Geometry: final body of the model. Coordinates: model frame, mm. Face numbers are marked on the shaded views. A direction names the side the tool comes from. Give positions to 0.01 mm unless a question says otherwise; leave off trailing zeros. Write each loop counter-clockwise with the first axis right and the second up, starting at its lowest first coordinate (ties: lowest second). Pieces come first, ordered by that corner, then holes. Notation, with made-up numbers: M 85,-23 L 141,-23 A18 ccw 141,-14 Z; hole C 17,35 d10. An arc over 180 degrees is marked long. One line per question, with ' | ' between items.
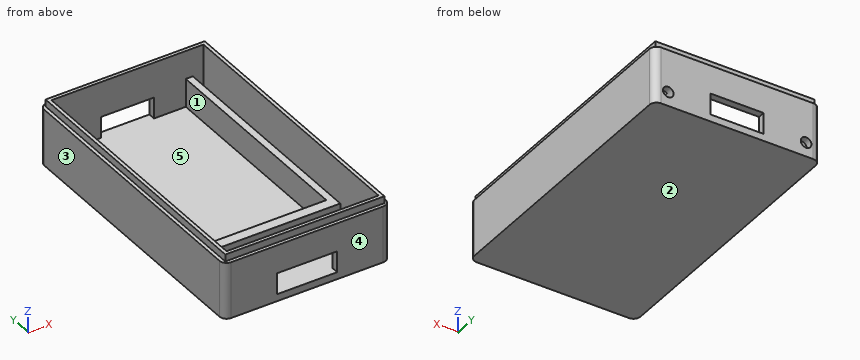
from build123d import *

# Parameters (mm, degrees)
SKETCH1_W           = 47
SKETCH1_H           = 80
BOSS_EXTRUDE1_DEPTH = 18
SKETCH2_W           = 43
SKETCH2_H           = 76
CUT_EXTRUDE1_DEPTH  = 16
BOSS_EXTRUDE2_DEPTH = 8
SKETCH6_W           = 15
SKETCH6_H           = 6
CUT_EXTRUDE4_DEPTH  = 11
SKETCH8_W           = 47
SKETCH8_H           = 80
SKETCH8_W_2         = 45
SKETCH8_H_2         = 78
CUT_EXTRUDE5_DEPTH  = 2
SKETCH9_R           = 1.5
CUT_EXTRUDE6_DEPTH  = 10
SKETCH11_W          = 17
SKETCH11_H          = 6
CUT_EXTRUDE9_DEPTH  = 10
FILLET4_R           = 2


with BuildPart() as part:
    # Sketch1 → Boss-Extrude1 (new body)
    with BuildSketch(Plane.XY):
        Rectangle(SKETCH1_W, SKETCH1_H)
    extrude(amount=BOSS_EXTRUDE1_DEPTH)

    # Sketch2 → Cut-Extrude1 (cut)
    with BuildSketch(Plane.XY.offset(18)):
        Rectangle(SKETCH2_W, SKETCH2_H)
    extrude(amount=-CUT_EXTRUDE1_DEPTH, mode=Mode.SUBTRACT)

    # Sketch3 → Boss-Extrude2 (add)
    with BuildSketch(Plane.XY.offset(2)):
        Polygon((-18.5, 38), (-16.5, 38), (-16.5, -23), (16.5, -23), (16.5, 38), (18.5, 38), (18.5, -26), (-18.5, -26), align=None)
    extrude(amount=BOSS_EXTRUDE2_DEPTH)

    # Sketch6 → Cut-Extrude4 (cut)
    with BuildSketch(Plane.XZ.offset(-38)):
        with Locations((0, 5)):
            Rectangle(SKETCH6_W, SKETCH6_H)
    extrude(amount=-CUT_EXTRUDE4_DEPTH, mode=Mode.SUBTRACT)

    # Sketch8 → Cut-Extrude5 (cut)
    with BuildSketch(Plane.XY.offset(18)):
        Rectangle(SKETCH8_W, SKETCH8_H)
        Rectangle(SKETCH8_W_2, SKETCH8_H_2, mode=Mode.SUBTRACT)
    extrude(amount=-CUT_EXTRUDE5_DEPTH, mode=Mode.SUBTRACT)

    # Sketch9 → Cut-Extrude6 (cut)
    with BuildSketch(Plane(origin=(0, 40, 0), x_dir=(1, 0, 0), z_dir=(0, 1, 0))):
        with Locations(Location((-19.5, -4, 0), (0, 0, 270))):
            Circle(SKETCH9_R)
        with Locations(Location((19.5, -4, 0), (0, 0, 228.189685104))):
            Circle(SKETCH9_R)
    extrude(amount=-CUT_EXTRUDE6_DEPTH, mode=Mode.SUBTRACT)

    # Sketch11 → Cut-Extrude9 (cut)
    with BuildSketch(Plane(origin=(0, -38, 0), x_dir=(1, 0, 0), z_dir=(0, 1, 0))):
        with Locations((0, -5)):
            Rectangle(SKETCH11_W, SKETCH11_H)
    extrude(amount=-CUT_EXTRUDE9_DEPTH, mode=Mode.SUBTRACT)

    # Fillet4
    fillet4_edges = [part.edges().sort_by_distance(p)[0] for p in [
        (23.5, -40, 8),
        (-23.5, -40, 8),
        (-23.5, 40, 8),
        (23.5, 40, 8),
    ]]
    fillet(fillet4_edges, radius=FILLET4_R)


solid = part.part
(1) Cut plane C-C, the plane y = 16. Return loops of the section in (x, z).
Working result:
outline: M -23.5,0 L 23.5,0 L 23.5,16 L 22.5,16 L 22.5,18 L 21.5,18 L 21.5,2 L 18.5,2 L 18.5,10 L 16.5,10 L 16.5,2 L -16.5,2 L -16.5,10 L -18.5,10 L -18.5,2 L -21.5,2 L -21.5,18 L -22.5,18 L -22.5,16 L -23.5,16 Z
(2) Cut plane B-B, the plane z = 12.5. Return loops of the section in (x, y), then the cut area to 3 significant figures.
Working result:
outline: M -23.5,-38 A2 ccw -21.5,-40 L 21.5,-40 A2 ccw 23.5,-38 L 23.5,38 A2 ccw 21.5,40 L -21.5,40 A2 ccw -23.5,38 Z; hole M -21.5,-38 L 21.5,-38 L 21.5,38 L -21.5,38 Z | area: 489 mm^2
(3) Set-up query: the marked faces 1 and 2. Return all of +Z, -Z, +X, -X, +Y, -Y with unobstructed straight access to the full face (end or side cutting, diameter ignored); none if empty.
Working result:
face 1: +Z | face 2: -Z, +X, -X, +Y, -Y
(4) First-contact query: P1, Ø3, axis at x = 3.5, z = 3, coming from the -Y side; P2, Ø1.6, axis at x = 8, z = 17, coming from the -Y side; P3, Ø1.6, axis at y = 39.5, z = 4, coming from the -X side; P4, Ø0.6, axis at y = 8.5, z = 17, coming from the +X side. Flat tips, straight axial feed; report the tip coordinate or a pass-through.
Working result:
P1: stops at y = -40 | P2: stops at y = -39 | P3: stops at x = -23.37 | P4: stops at x = 22.5
(5) Cut plane D-D, the plane x = -19.5. Return loops of the section in (y, z), then the cut area to 3 significant figures.
Working result:
outline: M -40,0 L 40,0 L 40,2.5 L 38,2.5 L 38,2 L -38,2 L -38,18 L -39,18 L -39,16 L -40,16 Z; M 38,5.5 L 40,5.5 L 40,16 L 39,16 L 39,18 L 38,18 Z | area: 214 mm^2
(6) Draft query along Y for the marked faces 3, 4 and 5. Return one class per face: released by +Y, released by -Y, zero draft, split by the parting line, or undercut.
Working result:
face 3: zero draft | face 4: released by -Y | face 5: undercut
(7) Material intervals for L1, parallel to X at y = 33.75, z = 4; L2, parallel to X at y = -15, z = 2.75; L3, parallel to Y at x = 14, z = 3.75, sorted ascending. Write a range as [from, to].
Working result:
L1: x = [-23.5, -21.5], [-18, -16.5], [16.5, 18], [21.5, 23.5] | L2: x = [-23.5, -21.5], [-18.5, -16.5], [16.5, 18.5], [21.5, 23.5] | L3: y = [-40, -38], [-26, -23], [38, 40]
(8) Cut plane A-A, the plane x = -6. Return loops of the section in (y, z), then the cut area to 3 significant figures.
Working result:
outline: M -40,0 L 40,0 L 40,2 L -23,2 L -23,10 L -26,10 L -26,2 L -40,2 Z; M -40,8 L -38,8 L -38,18 L -39,18 L -39,16 L -40,16 Z; M 38,8 L 40,8 L 40,16 L 39,16 L 39,18 L 38,18 Z | area: 220 mm^2
